Autodesk Inventor part; units mm, degrees
ref_plane "YZ Plane" through (0, 0, 0) normal (1, 0, 0) x (0, 1, 0)
ref_plane "XZ Plane" through (0, 0, 0) normal (0, 1, 0) x (-1, 0, 0)
ref_plane "XY Plane" through (0, 0, 0) normal (0, 0, 1) x (1, 0, 0)
sketch "Sketch1" plane through (0, 0, 0) normal (0, 1, 0) x (-1, 0, 0)
  circle A0 centre (0, 0) radius 3.5
  circle A1 centre (0, 0) radius 2.25
  circle A2 centre (0, 0) radius 1.4
  line L0 (0, 0) -> (-1.4, 0)
  line L1 (-1.4, 0) -> (-1.4, -1.4)
  line L2 (-1.4, -1.4) -> (0, -1.4)
  line L3 (0, -1.4) -> (0, 0)
  line L4 (-1.4, -1.4) -> (7.6159, -1.4)
  line L5 (7.6159, -1.4) -> (7.6159, 1.4)
  line L6 (7.6159, 1.4) -> (-1.4, 1.4)
  line L7 (-1.4, 1.4) -> (-1.4, -1.4)
  point P0 (0, 1.4)
  point P1 (3.2078, 1.4)
  point P2 (3.2078, -1.4)
  point P3 (1.7614, 1.4)
  point P4 (1.7614, -1.4)
  dimension "d0" = 7
  dimension "d1" = 4.5
  dimension "d6" = 2.8
extrude "Extrusion1" add sketch "Sketch1" against normal blind 110 contours L6 A1 L4 A0 | L6 L7 L1 L2 L4 A1 | A2 L7 L6 | L2 L1 A2 picked at (2.5783, 1.6484)
extrude "Extrusion2" add sketch "Sketch1" along normal blind 15 contours L6 L7 L1 L2 L4 A1 | A2 L7 L6 | L2 L1 A2
sketch "Sketch2" plane through (0, -110, 0) normal (0, -1, 0) x (1, 0, 0)
  circle A0 centre (0, 0) radius 4.75
  circle A1 centre (0, 0) radius 7.5
  arc A2 (-3.2078, -1.4) -> (-3.2078, 1.4) centre (0, 0) ccw
  line L0 (-3.2078, 1.4) -> (0, 1.4)
  arc A3 (0, -1.4) -> (0, 1.4) centre (0, 0) ccw
  line L1 (0, -1.4) -> (-3.2078, -1.4)
  line L2 (1.4, -1.4) -> (-7.6159, -1.4)
  line L3 (-7.6159, 1.4) -> (1.4, 1.4)
  point P0 (-4.539, 1.4)
  point P1 (-4.539, -1.4)
  point P2 (-7.3682, 1.4)
  point P3 (-7.3682, -1.4)
  dimension "d7" = 9.5
  dimension "d8" = 15
extrude "Extrusion3" add sketch "Sketch2" against normal blind 25 contours A0 L2 A2 L3
extrude "Extrusion4" add sketch "Sketch2" along normal blind 10 contours A0 L2 A2 L3 | A0 L3 A1 L2 | A2 L1 A3 L0 picked at (6.4638, 0.9807)
properties part number "Norhof wire channel top"
The listing builds one solid part. Answer for the finished solid, in the listing's coordinates (mm). A direction names the side the tool comes from. Coordinates: 2 decimals unless noted, no trailing zeros. Order: outer loops, then holes, each group sorted by start corner. A loop starts at its lowest first (then second) coordinate and runs counter-clockwise, first axis right, second up. Notation, with made-up numbers: (88.5, -33.75) -> (136.5, -33.75) arc R25 cw to (136.5, -2.75) -> close; hole circle Ø10 at (-15.5, 38). An arc over 180 degrees is marked (long way). Answer in a Markdown table with one row per item. Add a question column.
Item 1: Each of these flat-tipped pins is pushed along its axis until it touches: P1, Ø8, axis at x = -3, y = -73.5, coming from the -Z side; P2, Ø5, axis at x = -3, y = -20, coming from the +Z side; P3, Ø8, axis at y = -86.5, z = 3, coming from the +X side. Where does it stop, or does it pass through?
Item 2: Determine the mould class of faces 4 (the face through (-2, -68, 1.4)), 5 (the face through (7.494, -114.93, 0.31)), 6 (the face through (2, 0, -2)) for opening direction Z: +Z half, -Z half, draft (parallel to the pull), parting line (faces both ways), or undercut.
Item 3: Find section A-A (z = 0). Write down the section's boundary in (x, y), then the cut area to 3 significant figures.
Item 4: Find section C-C (z = -6). Write down the section's boundary in (x, y).
Item 5: Find the intervals of material crossed by L1, parallel to Y at x = 1, z = -5.75; L2, parallel to Y at x = -2.25, z = 2; L3, parallel to Z at x = -3.5, y = -97, in increasing order. Write a range as from..to.
Item 6: Which of the six approach directions +Z, -Z, +X, -X, +Y, -Y give full straight-line access (tool end or side, diameter ignored) to faces 1 (the face through (2.25, 7.4, -0.08)), 2 (the face through (-2, -68, -1.4)), 3 (the face through (2, -120, 0))?
Item 7: Find section B-B (y = -92). Write down the section's boundary in (x, z), then the cut area to 3 significant figures.
Result set:
| question | item | result |
|---|---|---|
| 1 | P1 | stops at z = -3.5 |
| 1 | P2 | stops at z = 3.46 |
| 1 | P3 | stops at x = 4.75 |
| 2 | face 4 | undercut |
| 2 | face 5 | parting line |
| 2 | face 6 | draft |
| 3 | outline | (1.4, -120) -> (7.5, -120) -> (7.5, -110) -> (4.75, -110) -> (4.75, -85) -> (3.5, -85) -> (3.5, 0) -> (2.25, 0) -> (2.25, 15) -> (1.4, 15) -> close |
| 3 | area | 336 mm² |
| 4 | outline | (-4.5, -120) -> (4.5, -120) -> (4.5, -110) -> (-4.5, -110) -> close |
| 5 | L1 | y = -120..-110 |
| 5 | L2 | y = -120..0 |
| 5 | L3 | z = -3.21..-1.4, 1.4..3.21 |
| 6 | face 1 | +Y |
| 6 | face 2 | -X, +Y, -Y |
| 6 | face 3 | +Z, -Z, +X, -X, -Y |
| 7 | outline | (-4.54, -1.4) arc R4.75 ccw (long way) to (-4.54, 1.4) -> (0, 1.4) arc R1.4 cw to (0, -1.4) -> close |
| 7 | area | 54.7 mm² |
